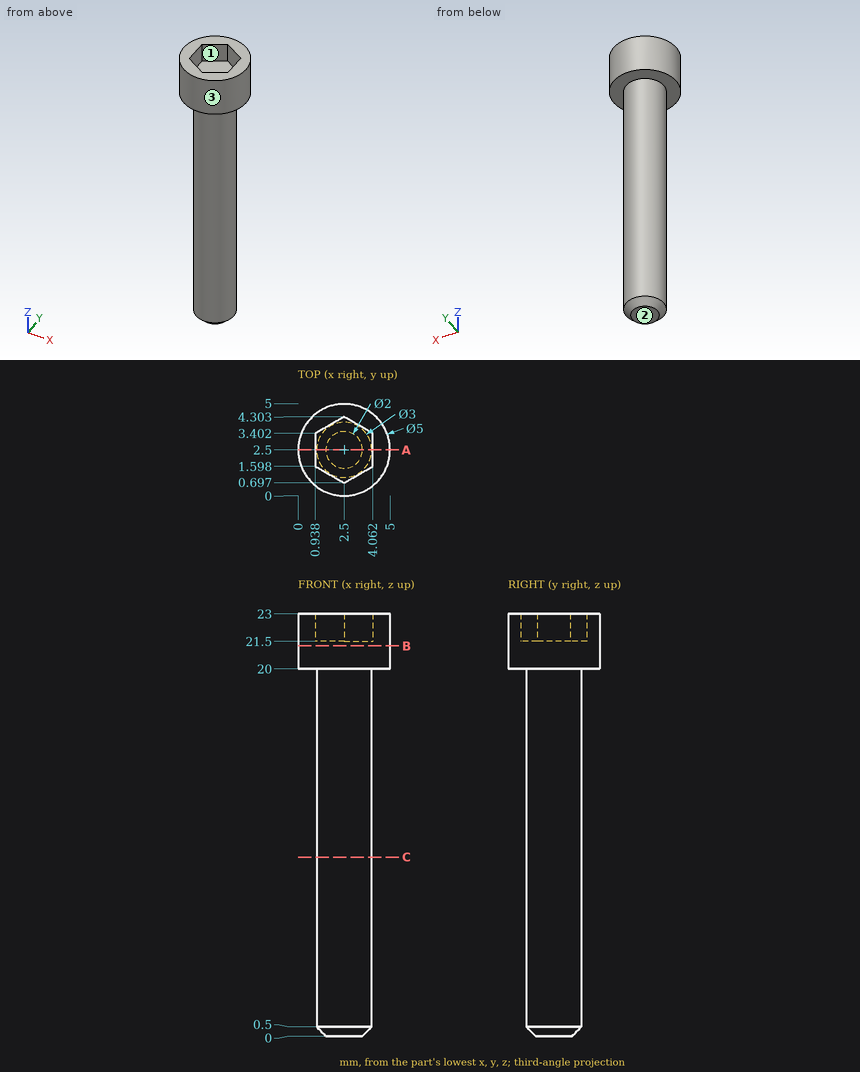
Check sheet for the drawn part. Datum: minimum x, y, z corner. Units: mm. Coordinates: 2 decimals unless noted, no trailing zeros. Write each loop counter-clockwise with the first axis right and the second up, starting at its lowest first coordinate (ties: lowest second). Pieces come first, ordered by that corner, then holes. Notation, with made-up numbers: (-17, 75.25) - (35, 75.25) arc R15 ccw to (35, 81.25) - close; hole circle Ø9 at (31, 18.25). An arc over 180 degrees is marked (long way). Answer as a JSON object with one key per item and string values.
(1) Cross-section at B-B on z = 21.25. Record the cut outline in (x, y), plus the area to 3 significant figures.
Report:
{"outline": "circle Ø5 at (2.5, 2.5)", "area": "19.6 mm^2"}
(2) Gauge pin test, flat ends, axial feed: pin 1 Ø3 at (y, z) = (2, 13.5) entering from -X; pin 2 Ø0.9 at (x, y) = (2.5, 3) entering from +Z. Record the tip position at first contact, or that the pin passes through.
Report:
{"pin 1": "x = 1", "pin 2": "z = 21.5"}
(3) Thickness scan on line 1 along Y through (x, z) = (2.45, 3); line 2 along Z through (x, y) = (2.2, 2.7); line 3 along Y through (x, z) = (3.7, 5.5). Record the ranges inside material, lowest first.
Report:
{"line 1": "1 to 4", "line 2": "0 to 21.5", "line 3": "1.6 to 3.4"}
(4) Mould release check, pull along X, two halves, no side actions. Record for the marked faces 1, 2 and 3: pulls with the +X half, pulls with the -X half, needs draft (parallel to the pull), parting line crosses it, or undercut.
Report:
{"face 1": "undercut", "face 2": "needs draft", "face 3": "parting line crosses it"}
(5) Cross-section at A-A on y = 2.5. Record the cut outline in (x, z).
Report:
{"outline": "(0, 20) - (1, 20) - (1, 0.5) - (1.5, 0) - (3.5, 0) - (4, 0.5) - (4, 20) - (5, 20) - (5, 23) - (4.06, 23) - (4.06, 21.5) - (0.94, 21.5) - (0.94, 23) - (0, 23) - close"}
(6) Cross-section at C-C on z = 9.75. Record the cut outline in (x, y).
Report:
{"outline": "circle Ø3 at (2.5, 2.5)"}
